Read the model definition and answer for the solid it produces. Units are mm, in the model's axes. A direction names the side the tool comes from. Coordinates: 2 decimals unless noted, no trailing zeros. Loops run counter-clockwise (first coordinate to the right, second up) from the corner with the lowest first, then second, coordinate; pieces in that order, holes last. Notation, with made-up numbers: M 18,70 L 37,70 A23 ccw 37,78 Z; hole C 29.5,13.5 d7. An arc over 180 degrees is marked long. One line per item, written item: value. Start each with the question number.
1. For faces 5 (the face through (-62.051, 1.351, 1.528)), 6 (the face through (-3.804, -10.689, 94.015)), determine the directions among +Z, -Z, +X, -X, +Y, -Y from which every point of the face is accessible in a straight line to the end or side of a thin tool.
2. Consider probe 1 along Z at (x, y) = (0, 18); probe 2 along Z at (x, y) = (-1.5, 79.5); probe 3 along Y at (x, z) = (12, 90). Determine where each line is inside the solid, lowest interval first.
3. The part is cut by section B-B (y = -55.5). Write down the section's boundary in (x, z), then the cut area to 3 significant figures.
4. A flat-ended cylindrical pin translates along its axis: pin 1 (8 mm diameter, centred on x = -1.5, z = 92, fed in from -Y). Find the tip coordinate at first contact, or state that the pin passes through.
5. The part is cut by section A-A (x = 0). Write down the section's boundary in (y, z).
6. The part is cut by section C-C (z = 60). Write down the section's boundary in (x, y), then the cut area to 3 significant figures.
7. Determine the mould class of faces 1 (the face through (0.818, 100.151, 1.528)), 2 (the face through (0, 82.804, 65)), 3 (the face through (62.051, 1.351, 125.472)), 4 (the face through (12, -101.6, 37)) for opening direction Z: +Z half, -Z half, draft (parallel to the pull), parting line (faces both ways), or undercut.
```python
from build123d import *

# Parameters (mm, degrees)
F0_W     = 127
F0_H     = 203.2
F1_DEPTH = 127
F2_R     = 5.08
F3_R     = 29.219894
F4_DEPTH = 184.404


with BuildPart() as f1:
    # F0 (on Top) → F1 (new body)
    with BuildSketch(Plane.XY):
        Rectangle(F0_W, F0_H)
    extrude(amount=F1_DEPTH)

    # F2
    f2_edges = [f1.edges().sort_by_distance(p)[0] for p in [
        (0, 101.6, 127),
        (-63.5, 0, 127),
        (0, -101.6, 127),
        (63.5, 0, 127),
        (-63.5, -101.6, 63.5),
        (63.5, -101.6, 63.5),
        (0, -101.6, 0),
        (63.5, 101.6, 63.5),
        (63.5, 0, 0),
        (-63.5, 101.6, 63.5),
        (0, 101.6, 0),
        (-63.5, 0, 0),
    ]]
    fillet(f2_edges, radius=F2_R)

    # F3 (on face) → F4 (cut)
    with BuildSketch(Plane.XZ.offset(101.6)):
        with Locations((0, 65.043747)):
            Circle(F3_R)
    extrude(amount=-F4_DEPTH, mode=Mode.SUBTRACT)


solid = f1.part
```
Answer block:
1. face 5: -Z, -X, +Y, -Y
1. face 6: -Y
2. probe 1: z = 0 to 35.82, 94.26 to 127
2. probe 2: z = 0 to 35.86, 94.23 to 127
2. probe 3: y = 82.8 to 101.6
3. outline: M -63.5,5.08 A5.08 ccw -58.42,0 L 58.42,0 A5.08 ccw 63.5,5.08 L 63.5,121.92 A5.08 ccw 58.42,127 L -58.42,127 A5.08 ccw -63.5,121.92 Z; hole C 0,65.04 d58.44
3. area: 13,400 mm2
4. pin 1: stops at y = -101.6
5. outline: M -101.6,5.08 A5.08 ccw -96.52,0 L 96.52,0 A5.08 ccw 101.6,5.08 L 101.6,121.92 A5.08 ccw 96.52,127 L -96.52,127 A5.08 ccw -101.6,121.92 L -101.6,94.26 L 82.8,94.26 L 82.8,35.82 L -101.6,35.82 Z
6. outline: M -63.5,-96.52 A5.08 ccw -58.42,-101.6 L -28.78,-101.6 L -28.78,82.8 L 28.78,82.8 L 28.78,-101.6 L 58.42,-101.6 A5.08 ccw 63.5,-96.52 L 63.5,96.52 A5.08 ccw 58.42,101.6 L -58.42,101.6 A5.08 ccw -63.5,96.52 Z
6. area: 15,200 mm2
7. face 1: -Z half
7. face 2: undercut
7. face 3: +Z half
7. face 4: draft
